Part model, mm, in its own coordinate system. A direction names the side the tool comes from. Round coordinates to 2 decimals unless told otherwise and drop trailing zeros. Loops run counter-clockwise (first coordinate to the right, second up) from the corner with the lowest first, then second, coordinate; pieces in that order, holes last.
from build123d import *

# Parameters (mm, degrees)
SKETCH_1_R          = 4.9
EXTRUDE_1_DEPTH     = 10
EXTRUDE_2_DEPTH     = 20
SKETCH_3_R          = 5
EXTRUDE_3_DEPTH     = 20
CHAMFER_1_SIZE      = 2
CUT_EXTRUDE_1_DEPTH = 1
SKETCH_5_W          = 112.212059924
SKETCH_5_H          = 221.512042167
CUT_EXTRUDE_2_DEPTH = 23
CUT_EXTRUDE_3_DEPTH = 14


with BuildPart() as part:
    # 草图1 → 凸台-拉伸1 (new body)
    with BuildSketch(Plane(origin=(0, 0, 0), x_dir=(0, 0, -1), z_dir=(1, 0, 0))):
        Circle(SKETCH_1_R)
    extrude(amount=EXTRUDE_1_DEPTH)

    # 草图2 → 凸台-拉伸2 (add)
    with BuildSketch(Plane(origin=(10, 0, 0), x_dir=(0, 0, -1), z_dir=(1, 0, 0))):
        with BuildLine():
            Line((15, 0), (15, -75))
            ThreePointArc((15, -75), (0, -90), (-15, -75))
            Line((-15, -75), (-15, 0))
            ThreePointArc((-15, 0), (0, 15), (15, 0))
        make_face()
    extrude(amount=EXTRUDE_2_DEPTH)

    # 草图3 → 凸台-拉伸3 (add)
    with BuildSketch(Plane.ZY.offset(-10)):
        with Locations(Location((0, -75, 0), (0, 0, 180))):
            Circle(SKETCH_3_R)
    extrude(amount=EXTRUDE_3_DEPTH)

    # 倒角1
    chamfer_1_edges = [part.edges().sort_by_distance(p)[0] for p in [
        (10, -37.5, 15),
        (10, -90, 0),
        (30, -37.5, -15),
        (10, 15, 0),
        (30, -37.5, 15),
        (30, -90, 0),
        (30, 15, 0),
        (10, -37.5, -15),
    ]]
    chamfer(chamfer_1_edges, length=CHAMFER_1_SIZE)

    # 草图4 → 切除-拉伸1 (cut)
    with BuildSketch(Plane(origin=(30, 0, 0), x_dir=(0, 0, -1), z_dir=(1, 0, 0))):
        with BuildLine():
            Line((6.835634275, 0), (6.835634275, -75))
            ThreePointArc((6.835634275, -75), (0, -81.835634275), (-6.835634275, -75))
            Line((-6.835634275, -75), (-6.835634275, 0))
            ThreePointArc((-6.835634275, 0), (0, 6.835634275), (6.835634275, 0))
        make_face()
    extrude(amount=-CUT_EXTRUDE_1_DEPTH, mode=Mode.SUBTRACT)

    # 草图5 → 切除-拉伸2 (cut)
    with BuildSketch(Plane.ZY.offset(10)):
        with Locations((-34.944932156, -94.819395662)):
            Rectangle(SKETCH_5_W, SKETCH_5_H)
    extrude(amount=-CUT_EXTRUDE_2_DEPTH, mode=Mode.SUBTRACT)

    # 草图6 → 切除-拉伸3 (cut)
    with BuildSketch(Plane.ZY.offset(-13)):
        with BuildLine():
            Line((13, 0), (13, -75))
            ThreePointArc((13, -75), (0, -88), (-13, -75))
            Line((-13, -75), (-13, 0))
            ThreePointArc((-13, 0), (0, 13), (13, 0))
        make_face()
    extrude(amount=-CUT_EXTRUDE_3_DEPTH, mode=Mode.SUBTRACT)


solid = part.part
1) Wall check: line 1 along Z through (x, y) = (19.75, -75); line 2 along X through (y, z) = (-27.5, 12.5); line 3 along Y through (x, z) = (24.5, 8). Give the ranges that are in metal, low to high.
Values:
line 1: z = -15 to -13, 13 to 15
line 2: x = 27 to 30
line 3: y = -87.69 to -85.25, 10.25 to 12.69
2) Slice it at C-C, the plane y = -14.5. Give the cut face in (x, z), then the cut area to 3 significant figures.
Values:
outline: (13, -15) - (28, -15) - (30, -13) - (30, -6.84) - (29, -6.84) - (29, 6.84) - (30, 6.84) - (30, 13) - (28, 15) - (13, 15) - (13, 13) - (27, 13) - (27, -13) - (13, -13) - close
area: 128 mm2
3) Tool access for faces 1 (the face through (29, -37, 0)), 2 (the face through (30, -37, -9)), 3 (the face through (20, -38, -13)): list every direction of +Z, -Z, +X, -X, +Y, -Y with a clear straight run to the whole face (end or side of a thin tool).
Values:
face 1: +X
face 2: +Z, -Z, +X, +Y, -Y
face 3: -X
4) Drop flat-ended pins along their axis: pin 1 Ø6 at (x, z) = (16.5, -7.5) entering from -Y; pin 2 Ø6 at (y, z) = (-42, 7.5) entering from -X; pin 3 Ø0.8 at (x, y) = (29.5, -43.5) entering from +Z. Give the stop position or say it passes through.
Values:
pin 1: stops at y = -89.31
pin 2: stops at x = 27
pin 3: stops at z = 13.9
5) Slice it at A-A, the plane x = 22.75. Give the cut face in (y, z).
Values:
outline: (-75, -15) - (0, -15) arc R15 ccw to (0, 15) - (-75, 15) arc R15 ccw to start; hole (-75, -13) - (0, -13) arc R13 ccw to (0, 13) - (-75, 13) arc R13 ccw to start
6) Slice it at B-B, the plane z = 0. Give the cut face in (x, y), then the cut area to 3 significant figures.
Values:
outline: (13, -90) - (28, -90) - (30, -88) - (30, -81.84) - (29, -81.84) - (29, 6.84) - (30, 6.84) - (30, 13) - (28, 15) - (13, 15) - (13, 13) - (27, 13) - (27, -88) - (13, -88) - close
area: 278 mm2
7) Mould opens along Y. For faces 4 (the face through (20, -37, -15)), 5 (the face through (29.507, -81.834, -0.15)), 6 (the face through (20, -90, 0)), 7 (the face through (20, -88, 0)) say: released by +Y, released by -Y, zero draft, split by the parting line, or undercut.
Values:
face 4: zero draft
face 5: undercut
face 6: released by -Y
face 7: undercut
